Autodesk Inventor part; units mm, degrees
ref_plane "YZ Plane" through (0, 0, 0) normal (1, 0, 0) x (0, 1, 0)
ref_plane "XZ Plane" through (0, 0, 0) normal (0, 1, 0) x (-1, 0, 0)
ref_plane "XY Plane" through (0, 0, 0) normal (0, 0, 1) x (1, 0, 0)
sketch "Sketch1" plane through (0, 0, 0) normal (0, 1, 0) x (-1, 0, 0)
  line L0 (0, 40) -> (-35, 40)
  line L1 (-35, -40) -> (0, -40)
  arc A0 (0, -40) -> (0, 40) centre (0, 0) ccw
  line L2 (-35, 43) -> (0, 43)
  arc A1 (0, -43) -> (0, 43) centre (0, 0) ccw
  line L3 (0, -43) -> (-35, -43)
  line L4 (-35, 43) -> (-40, 43)
  line L5 (-40, 43) -> (-40, 40)
  line L6 (-40, 40) -> (-35, 40)
  line L7 (-35, -40) -> (-40, -40)
  line L8 (-40, -40) -> (-40, -43)
  line L9 (-40, -43) -> (-35, -43)
  dimension "d7" = 3
extrude "Extrusion1" add sketch "Sketch1" along normal blind 80
sketch "Sketch2" plane through (0, 80, 0) normal (0, 1, 0) x (1, 0, 0)
  line L0 (40, 43) -> (0, 43)
  arc A0 (0, 43) -> (0, -43) centre (0, 0) ccw
  line L1 (0, -43) -> (40, -43)
  line L2 (40, -43) -> (43, -43)
  line L3 (43, -43) -> (43, -40)
  line L4 (0, 40) -> (40, 40)
  line L5 (43, 40) -> (43, 43)
  line L6 (43, 43) -> (40, 43)
  line L7 (43, -40) -> (43, 40)
extrude "Extrusion2" add sketch "Sketch2" along normal blind 3
sketch "Sketch3" plane through (0, 83, 0) normal (0, 1, 0) x (1, 0, 0)
  line L0 (43, -43) -> (43, 43)
  line L1 (43, 23.4737) -> (38.5, 23.4737)
  line L2 (38.5, 26.4737) -> (43, 26.4737)
  line L3 (43, 26.4737) -> (43, 23.4737)
  arc A0 (38.5, 26.4737) -> (38.5, 23.4737) centre (38.5, 24.9737) ccw
extrude "Extrusion3" cut sketch "Sketch3" against normal blind 3
fillet "Fillet1" radius 2 6 edges at (21.5, 83, 43) (21.5, 83, -43) (-43, 83, 0) (37, 83, -24.9737) (40.75, 83, -26.4737) (40.75, 83, -23.4737)
properties part number "Telo_3DPrint"
Design review of the part built by this model. Coordinates are the model's own, in mm. A direction names the side the tool comes from. Give positions to 0.01 mm unless a question says otherwise; leave off trailing zeros. Loops run counter-clockwise (first coordinate to the right, second up) from the corner with the lowest first, then second, coordinate; pieces in that order, holes last. Notation, with made-up numbers: (-32.5, 2.5) -> (-16.5, 2.5) arc R12 ccw to (-16.5, 22.5) -> close; hole circle Ø6 at (13.25, 45). An arc over 180 degrees is marked (long way). One line per question, with ' | ' between items. Start each with the question number.
(1) Insertion check: P1, Ø8, axis at y = 43.5, z = 13.5, coming from the +X side; P2, Ø0.9, axis at y = 45.5, z = -41, coming from the +X side; P3, Ø1, axis at y = 17.5, z = -32.5, coming from the +X side. Each pin has a flat end and moves straight along its axis. Give the tip position at first contact, or say it passes through.
(2) For faces 4 (the face through (40, 39, 42)), 5 (the face through (20, 39, 40)), 6 (the face through (0, 83, -1)), list the 3-axis set-ups (+Z, -Z, +X, -X, +Y, -Y) from which the entire face can be reached by the end or side of a thin tool; tool diameter is ignored.
(3) Draft analysis for pull direction Z (two halves, no side actions). For faces 1 (the face through (40, 39, -41)), 2 (the face through (-39.99, 39.44, 0.88)), 3 (the face through (16, 40, -43)), state which applies: +Z half, -Z half, draft (parallel to the pull), parting line (faces both ways), or undercut.
(4) We need section A-A (x = 33). State the section outline as (y, z) points, and give its area (3 significant figures).
(5) For line 1 (Z direction, x = 22, y = 12.5); line 2 (Y direction, x = -28, z = 10.5); line 3 (Z direction, x = -13, y = 28), list the stretches that pass through material, from the lowest coordinate up.
(6) We need section C-C (y = 64.5). State the section outline as (x, z) points, and give its area (3 significant figures).
(7) We need section B-B (z = 0). State the section outline as (x, y) points.
The answers:
1) P1: stops at x = -35.97 | P2: stops at x = 40 | P3: stops at x = -22.61
2) face 4: +Z, -Z, +X, -Y | face 5: +X, -Y | face 6: +Z, -Z, +X, -X, +Y
3) face 1: draft | face 2: undercut | face 3: -Z half
4) outline: (0, -43) -> (81, -43) arc R2 ccw to (83, -41) -> (83, 41) arc R2 ccw to (81, 43) -> (0, 43) -> (0, 40) -> (80, 40) -> (80, -40) -> (0, -40) -> close | area: 736 mm^2
5) line 1: z = -43 to -40, 40 to 43 | line 2: y = 80 to 83 | line 3: z = -40.99 to -37.83, 37.83 to 40.99
6) outline: (0, -43) -> (40, -43) -> (40, -40) -> (0, -40) arc R40 cw to (0, 40) -> (40, 40) -> (40, 43) -> (0, 43) arc R43 ccw to start | area: 631 mm^2
7) outline: (-43, 0) -> (-40, 0) -> (-40, 80) -> (43, 80) -> (43, 83) -> (-41, 83) arc R2 ccw to (-43, 81) -> close
